Design review of the part built by this model. Coordinates are the model's own, in mm. A direction names the side the tool comes from. Give positions to 0.01 mm unless a question says otherwise; leave off trailing zeros. Write each loop counter-clockwise with the first axis right and the second up, starting at its lowest first coordinate (ties: lowest second). Pieces come first, ordered by that corner, then holes. Notation, with made-up numbers: (69, 1.25) -> (117, 1.25) arc R35 cw to (117, 36.25) -> close; hole circle Ø7 at (21, 19.25). An arc over 180 degrees is marked (long way). Answer as a JSON object with one key per item and string values.
```python
from build123d import *

# Parameters (mm, degrees)
BOSS_EXTRUDE1_DEPTH = 4
SKETCH2_R           = 1.600000002
CUT_EXTRUDE1_DEPTH  = 57.058005673
SKETCH3_R           = 1.6
BOSS_EXTRUDE3_DEPTH = 4
SKETCH4_W           = 4
SKETCH4_H           = 30
BOSS_EXTRUDE4_DEPTH = 4


with BuildPart() as part:
    # Sketch1 → Boss-Extrude1 (new body)
    with BuildSketch(Plane.XY):
        Polygon((-10.5, -45.5), (-10.5, -24.5), (10.5, -24.5), (10.5, -45.5), (32.5, -45.5), (32.5, 45.5), (-32.5, 45.5), (-32.5, -45.5), align=None)
    extrude(amount=BOSS_EXTRUDE1_DEPTH)

    # Sketch2 → Cut-Extrude1 (cut, through all)
    with BuildSketch(Plane(origin=(0, 0, 0), x_dir=(-1, 0, 0), z_dir=(0, 0, -1))):
        with Locations((18.999999999, -35.500025949)):
            Circle(SKETCH2_R)
        with Locations((-1e-09, -16.500025949)):
            Circle(SKETCH2_R)
        with Locations((-19.000000001, -35.500025949)):
            Circle(SKETCH2_R)
    extrude(amount=-CUT_EXTRUDE1_DEPTH, mode=Mode.SUBTRACT)

    # Sketch3 → Boss-Extrude3 (add)
    # profile 1 of 4: a face of its own
    with BuildSketch(Plane(origin=(0, 0, 0), x_dir=(-1, 0, 0), z_dir=(0, 0, -1))):
        with BuildLine():
            Line((34.5, 38.5), (32.5, 38.5))
            Line((32.5, 38.5), (32.5, 32.5))
            Line((32.5, 32.5), (34.5, 32.5))
            ThreePointArc((34.5, 32.5), (37.5, 35.5), (34.5, 38.5))
        make_face()
        with Locations((34.5, 35.5)):
            Circle(SKETCH3_R, mode=Mode.SUBTRACT)
    # profile 2 of 4: a face of its own
    with BuildSketch(Plane(origin=(0, 0, 0), x_dir=(-1, 0, 0), z_dir=(0, 0, -1))):
        with BuildLine():
            Line((34.5, -32.5), (32.5, -32.5))
            Line((32.5, -32.5), (32.5, -38.5))
            Line((32.5, -38.5), (34.5, -38.5))
            ThreePointArc((34.5, -38.5), (37.5, -35.5), (34.5, -32.5))
        make_face()
        with Locations((34.5, -35.5)):
            Circle(SKETCH3_R, mode=Mode.SUBTRACT)
    # profile 3 of 4: a face of its own
    with BuildSketch(Plane(origin=(0, 0, 0), x_dir=(-1, 0, 0), z_dir=(0, 0, -1))):
        with BuildLine():
            Line((-34.5, -38.5), (-32.5, -38.5))
            Line((-32.5, -38.5), (-32.5, -32.5))
            Line((-32.5, -32.5), (-34.5, -32.5))
            ThreePointArc((-34.5, -32.5), (-37.5, -35.5), (-34.5, -38.5))
        make_face()
        with Locations((-34.5, -35.5)):
            Circle(SKETCH3_R, mode=Mode.SUBTRACT)
    # profile 4 of 4: a face of its own
    with BuildSketch(Plane(origin=(0, 0, 0), x_dir=(-1, 0, 0), z_dir=(0, 0, -1))):
        with BuildLine():
            Line((-34.5, 32.5), (-32.5, 32.5))
            Line((-32.5, 32.5), (-32.5, 38.5))
            Line((-32.5, 38.5), (-34.5, 38.5))
            ThreePointArc((-34.5, 38.5), (-37.5, 35.5), (-34.5, 32.5))
        make_face()
        with Locations((-34.5, 35.5)):
            Circle(SKETCH3_R, mode=Mode.SUBTRACT)
    extrude(amount=-BOSS_EXTRUDE3_DEPTH)

    # Sketch4 → Boss-Extrude4 (add)
    with BuildSketch(Plane(origin=(0, 0, 0), x_dir=(-1, 0, 0), z_dir=(0, 0, -1))):
        with Locations((34.5, 0)):
            Rectangle(SKETCH4_W, SKETCH4_H)
        with Locations((-34.5, 0)):
            Rectangle(SKETCH4_W, SKETCH4_H)
    extrude(amount=-BOSS_EXTRUDE4_DEPTH)


solid = part.part
```
(1) We need section A-A, the plane x = 0. State the section outline as (y, z) points, then the cut area to 3 significant figures.
Here are the results:
{"outline": "(-24.5, 0) -> (-18.1, 0) -> (-18.1, 4) -> (-24.5, 4) -> close; (-14.9, 0) -> (45.5, 0) -> (45.5, 4) -> (-14.9, 4) -> close", "area": "267 mm²"}
(2) For line 1 along Y through (x, z) = (-34.5, 0.9); line 2 along X through (y, z) = (-39.5, 3.05); line 3 along Y through (x, z) = (0, 2.8), list the stretches that pass through material, from the lowest coordinate up.
Here are the results:
{"line 1": "y = -38.5 to -37.1, -33.9 to -32.5, -15 to 15, 32.5 to 33.9, 37.1 to 38.5", "line 2": "x = -32.5 to -10.5, 10.5 to 32.5", "line 3": "y = -24.5 to -18.1, -14.9 to 45.5"}
(3) We need section C-C, the plane y = -19.5. State the section outline as (x, z) points.
Here are the results:
{"outline": "(-32.5, 0) -> (32.5, 0) -> (32.5, 4) -> (-32.5, 4) -> close"}
(4) The part is to be moulded in two halves that separate along Y. For faces 5 (the flat face through (-1, 1, 0)), 6 (the cylindrical face through (35.77, 34.53, 1.97)), 7 (the flat face through (-34, 38.5, 2)), say which applies: +Y half, -Y half, draft (parallel to the pull), parting line (faces both ways), or undercut.
Here are the results:
{"face 5": "draft", "face 6": "undercut", "face 7": "+Y half"}
(5) We need section B-B, the plane x = 19. State the section outline as (y, z) points, then the cut area to 3 significant figures.
Here are the results:
{"outline": "(-45.5, 0) -> (-37.1, 0) -> (-37.1, 4) -> (-45.5, 4) -> close; (-33.9, 0) -> (45.5, 0) -> (45.5, 4) -> (-33.9, 4) -> close", "area": "351 mm²"}
(6) For faces 1 (the flat face through (34, -38.5, 2)), 2 (the flat face through (35, 15, 2)), 3 (the flat face through (-32.5, -42, 2)), 4 (the flat face through (-34, 15, 2)), list the 3-axis set-ups (+Z, -Z, +X, -X, +Y, -Y) from which the entire face can be reached by the end or side of a thin tool; tool diameter is ignored.
Here are the results:
{"face 1": "+Z, -Z, +X, -Y", "face 2": "+Z, -Z, +X", "face 3": "+Z, -Z, -X, -Y", "face 4": "+Z, -Z, -X"}
(7) Clearance check with flat-ended pins moving along their axes: pin 1 (3 mm diameter, centred on x = -19, y = -35.5, fed in from +Z); pin 2 (1 mm diameter, centred on x = -33.5, z = 1, fed in from -Y); pin 3 (1.5 mm diameter, centred on y = -17, z = 3.5, fed in from +X); pin 4 (2 mm diameter, centred on y = 20.5, z = 1, fed in from -X). State where each tip first meets the part, or that it passes through.
Here are the results:
{"pin 1": "passes through", "pin 2": "stops at y = -38.5", "pin 3": "stops at x = 32.5", "pin 4": "stops at x = -32.5"}
(8) We need section D-D, the plane z = 2.25. Give the number of separate pieces and of enclosed holes in the cut face, then the cut area to 3 significant figures.
Here are the results:
{"separate pieces": "1", "enclosed holes": "7", "area": "5,760 mm²"}
